Source: CAD feature listing. Evaluate the final solid. Frame: model axes, mm. Face numbers are marked on the shaded views. A direction names the side the tool comes from. Coordinates: 2 decimals unless noted, no trailing zeros. Loops run counter-clockwise (first coordinate to the right, second up) from the corner with the lowest first, then second, coordinate; pieces in that order, holes last. Notation, with made-up numbers: (-24.5, -35.75) - (14.5, -35.75) arc R19 ccw to (14.5, -23.75) - close; hole circle Ø1 at (-9.5, -7.5). An arc over 180 degrees is marked (long way). Use one line per item in the form item = value. Start each with the question number.
from build123d import *

# Parameters (mm, degrees)
BOSS_EXTRUDE1_DEPTH            = 3
BOSS_EXTRUDE1_DEPTH_BACK       = 12.8
SKETCH1_W                      = 6
SKETCH1_H                      = 6
SKETCH10_W                     = 6
SKETCH10_H                     = 3.25
BOSS_EXTRUDE2_DEPTH            = 0.75
CUT_EXTRUDE2_DEPTH             = 0.1
CUT_EXTRUDE2_DEPTH_BACK        = 1
CUT_EXTRUDE3_DEPTH             = 5.5
CUT_EXTRUDE3_DEPTH_BACK        = 6.5
SKETCH5_R                      = 4.45
CUT_EXTRUDE4_REACH             = 40.346
SKETCH7_R                      = 0.525
CUT_EXTRUDE4_DIRECTION_2_REACH = 40.346
SKETCH8_W                      = 3
SKETCH8_H                      = 6.75
CUT_EXTRUDE5_DEPTH             = 1
FILLET1_R                      = 3.5
FILLET1_R_2                    = 2.5
CUT_EXTRUDE7_DEPTH             = 39.676090947


with BuildPart() as part:
    # Sketch1 → Boss-Extrude1 (new, two sides: drawn at the far end of the back side and taken through both)
    with BuildSketch(Plane.XY.offset(-BOSS_EXTRUDE1_DEPTH_BACK)):
        with Locations((122, -33)):
            Rectangle(SKETCH1_W, SKETCH1_H)
    extrude(amount=BOSS_EXTRUDE1_DEPTH + BOSS_EXTRUDE1_DEPTH_BACK)

    # Sketch10 → Boss-Extrude2 (add)
    with BuildSketch(Plane(origin=(0, -30, 0), x_dir=(1, 0, 0), z_dir=(0, 1, 0))):
        with Locations((122, 11.175)):
            Rectangle(SKETCH10_W, SKETCH10_H)
    extrude(amount=BOSS_EXTRUDE2_DEPTH)

    # Sketch4 → Cut-Extrude2 (cut, two sides: drawn at the far end of the back side and taken through both)
    with BuildSketch(Plane.ZY.offset(-121.85).offset(-CUT_EXTRUDE2_DEPTH_BACK)):
        with BuildLine():
            Line((-11.776969868, -34.5), (-11.623346252, -34.5))
            ThreePointArc((-11.623346252, -34.5), (-10.835914556, -34.188123693), (-10.475580755, -33.421654477))
            Line((-10.475580755, -33.421654477), (-10.040343544, -26.45))
            Line((-10.040343544, -26.45), (-13.359649062, -26.45))
            Line((-13.359649062, -26.45), (-12.924738676, -33.421601422))
            ThreePointArc((-12.924738676, -33.421601422), (-12.564420934, -34.188105493), (-11.776969868, -34.5))
        make_face()
    extrude(amount=CUT_EXTRUDE2_DEPTH + CUT_EXTRUDE2_DEPTH_BACK, mode=Mode.SUBTRACT)

    # Sketch5 → Cut-Extrude3 (cut, two sides: drawn at the far end of the back side and taken through both)
    with BuildSketch(Plane(origin=(0, 0, -3.85), x_dir=(-1, 0, 0), z_dir=(0, 0, -1)).offset(-CUT_EXTRUDE3_DEPTH_BACK)):
        with Locations((-122.25, -26.35)):
            Circle(SKETCH5_R)
    extrude(amount=CUT_EXTRUDE3_DEPTH + CUT_EXTRUDE3_DEPTH_BACK, mode=Mode.SUBTRACT)

    # Cut-Extrude4: up to this face of the body (flat: up to its plane)
    cut_extrude4_end = Plane(part.part.faces().sort_by_distance((119, -32.915397223, -5.057298496))[0])
    # Sketch7 → Cut-Extrude4 (cut, up to the picked face)
    with BuildSketch(Plane(origin=(121.75, 0, 0), x_dir=(0, 0, -1), z_dir=(1, 0, 0)), mode=Mode.PRIVATE) as cut_extrude4_sk1:
        with Locations(Location((11.7, -33.35, 0), (0, 0, 90))):
            Circle(SKETCH7_R)
    cut_extrude4_tool1 = split(extrude(cut_extrude4_sk1.sketch, amount=-CUT_EXTRUDE4_REACH, mode=Mode.PRIVATE), bisect_by=cut_extrude4_end, keep=Keep.BOTH, mode=Mode.PRIVATE)
    # Sketch7 → Cut-Extrude4 (cut, up to the picked face)
    with BuildSketch(Plane(origin=(121.75, 0, 0), x_dir=(0, 0, -1), z_dir=(1, 0, 0)), mode=Mode.PRIVATE) as cut_extrude4_sk2:
        with Locations(Location((11.7, -30.35, 0), (0, 0, 90))):
            Circle(SKETCH7_R)
    cut_extrude4_tool2 = split(extrude(cut_extrude4_sk2.sketch, amount=-CUT_EXTRUDE4_REACH, mode=Mode.PRIVATE), bisect_by=cut_extrude4_end, keep=Keep.BOTH, mode=Mode.PRIVATE)
    add(cut_extrude4_tool1.solids().sort_by(Axis((121.75, -33.35, -11.7), (-1, 0, 0)))[0], mode=Mode.SUBTRACT)
    add(cut_extrude4_tool2.solids().sort_by(Axis((121.75, -30.35, -11.7), (-1, 0, 0)))[0], mode=Mode.SUBTRACT)

    # Cut-Extrude4 direction 2: up to this face of the body (flat: up to its plane)
    cut_extrude4_direction_2_end = Plane(part.part.faces().sort_by_distance((125, -32.915397223, -5.057298496))[0])
    # Sketch7 → Cut-Extrude4 direction 2 (cut, up to the picked face)
    with BuildSketch(Plane(origin=(121.75, 0, 0), x_dir=(0, 0, -1), z_dir=(1, 0, 0)), mode=Mode.PRIVATE) as cut_extrude4_direction_2_sk1:
        with Locations(Location((11.7, -33.35, 0), (0, 0, 90))):
            Circle(SKETCH7_R)
    cut_extrude4_direction_2_tool1 = split(extrude(cut_extrude4_direction_2_sk1.sketch, amount=CUT_EXTRUDE4_DIRECTION_2_REACH, mode=Mode.PRIVATE), bisect_by=cut_extrude4_direction_2_end, keep=Keep.BOTH, mode=Mode.PRIVATE)
    # Sketch7 → Cut-Extrude4 direction 2 (cut, up to the picked face)
    with BuildSketch(Plane(origin=(121.75, 0, 0), x_dir=(0, 0, -1), z_dir=(1, 0, 0)), mode=Mode.PRIVATE) as cut_extrude4_direction_2_sk2:
        with Locations(Location((11.7, -30.35, 0), (0, 0, 90))):
            Circle(SKETCH7_R)
    cut_extrude4_direction_2_tool2 = split(extrude(cut_extrude4_direction_2_sk2.sketch, amount=CUT_EXTRUDE4_DIRECTION_2_REACH, mode=Mode.PRIVATE), bisect_by=cut_extrude4_direction_2_end, keep=Keep.BOTH, mode=Mode.PRIVATE)
    add(cut_extrude4_direction_2_tool1.solids().sort_by(Axis((121.75, -33.35, -11.7), (1, 0, 0)))[0], mode=Mode.SUBTRACT)
    add(cut_extrude4_direction_2_tool2.solids().sort_by(Axis((121.75, -30.35, -11.7), (1, 0, 0)))[0], mode=Mode.SUBTRACT)

    # Sketch8 → Cut-Extrude5 (cut)
    with BuildSketch(Plane(origin=(125, 0, 0), x_dir=(0, 0, -1), z_dir=(1, 0, 0))):
        with Locations((11.3, -32.625)):
            Rectangle(SKETCH8_W, SKETCH8_H)
    extrude(amount=-CUT_EXTRUDE5_DEPTH, mode=Mode.SUBTRACT)

    # Fillet1
    # the kernel refuses this fillet: 3.5, 2.5 mm, written as the material it takes off along each edge
    with BuildSketch(Plane(origin=(132.75, -36, -12.8), x_dir=(0, 0, 1), z_dir=(-1, 0, 0))) as fillet1_piece_1:
        with BuildLine():
            CenterArc((FILLET1_R, FILLET1_R), FILLET1_R, 180, 90)
            Line((0, FILLET1_R), (0, 0))
            Line((0, 0), (FILLET1_R, 0))
        make_face()
    extrude(amount=22.5, mode=Mode.SUBTRACT)
    # the kernel refuses this fillet: 3.5, 2.5 mm, written as the material it takes off along each edge
    with BuildSketch(Plane(origin=(119, -23, -12.8), x_dir=(0, 0, 1), z_dir=(0, -1, 0))) as fillet1_2_piece_1:
        with BuildLine():
            CenterArc((FILLET1_R_2, -FILLET1_R_2), FILLET1_R_2, 90, 90)
            Line((0, -FILLET1_R_2), (0, 0))
            Line((0, 0), (FILLET1_R_2, 0))
        make_face()
    extrude(amount=15.75, mode=Mode.SUBTRACT)

    # Sketch12 → Cut-Extrude7 (cut, through all)
    with BuildSketch(Plane.ZY.offset(-119)):
        Polygon((-6.404787377, -36), (-12.404787377, -34.227808088), (-12.404787377, -36), align=None)
    extrude(amount=-CUT_EXTRUDE7_DEPTH, mode=Mode.SUBTRACT)


solid = part.part
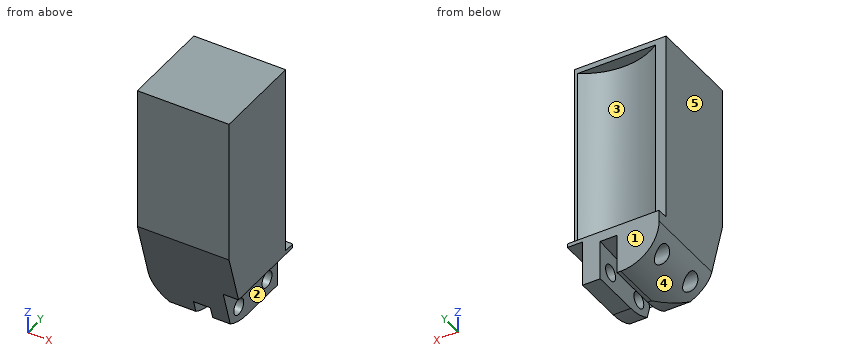
(1) Cut plane D-D, the plane z = -3.75. Output: boundary loops of the cut face in (x, y).
(2) Mould query, pull axis Z, two halves, no side actions, for the marked faces 3, 4 and 5. Classes: +Z half, -Z half, draft (parallel to the pull), parting line (faces both ways), or undercut.
(3) Access query for the marked faces 1 and 2. Directions: +Z, -Z, +X, -X, +Y, -Y. A direction counts if a zero-diameter tool reaches every point of the face in a straight line with its end or side. Return the directions, or none.
(4) Contact query for flat-ended pins moving along their axis: pin 1 (1.4 mm diameter, centred on y = -33.35, z = -11.7, fed in from +X); pin 2 (1.7 mm diameter, centred on y = -30.35, z = -11.7, fed in from -X); pin 3 (0.8 mm diameter, centred on y = -33.35, z = -11.7, fed in from +X); pin 4 (1 mm diameter, centred on x = 123.5, z = -8, fed in from +Y). Output: stop coordinate, or through.
(5) Cut plane B-B, the plane x = 120.25. Output: boundary loops of the cut face in (y, z) (3 decimals), plus the area to 3 significant figures.
(6) Material intervals for line 1 (Z direction, x = 123.6, y = -30.35) (3 decimals); line 2 (Y direction, x = 123.35, z = -11.7) (3 decimals); line 3 (Z direction, x = 120.65, y = -30.35) (3 decimals), sorted ascending.
(7) Cut plane A-A, the plane y = -33. Output: boundary loops of the cut face in (x, z), plus the area to 3 significant figures.
(8) Cut plane C-C, the plane y = -30.35. Output: boundary loops of the cut face in (x, z) (3 decimals).
Recorded:
q1.outline = (119, -36) - (125, -36) - (125, -30) - (124.8, -30) arc R4.45 cw to (119.7, -30) - (119, -30) - close
q2.face_3 = undercut
q2.face_4 = -Z half
q2.face_5 = draft
q3.face_1 = +Z, -Z, +X, -X, +Y
q3.face_2 = -Z, +X, +Y, -Y
q4.pin_1 = 124
q4.pin_2 = 119.06
q4.pin_3 = through
q4.pin_4 = -30.44
q5.outline = (-36, -6.405) - (-34.249, -12.331) arc R3.5 ccw to (-33.994, -12.465) - (-29.25, -12.465) - (-29.25, -9.55) - (-30, -9.55) - (-30, -9.35) - (-30.325, -9.35) - (-30.325, 2.65) - (-30, 2.65) - (-30, 3) - (-36, 3) - close; hole circle Ø1.05 at (-33.35, -11.7); hole circle Ø1.05 at (-30.35, -11.7)
q5.area = 83.9 mm²
q6.line_1 = -12.8 to -12.225, -11.175 to -9.35, 2.65 to 3
q6.line_2 = -34.436 to -33.875, -32.825 to -30.875, -29.825 to -29.25
q6.line_3 = -12.651 to -12.225, -11.175 to -9.35, 2.65 to 3
q7.outline = (119, -10.3) arc R2.5 ccw to (119.21, -11.31) - (121.75, -11.31) - (121.75, -10.45) - (122.85, -10.45) - (122.85, -11.31) - (124, -11.31) - (124, -9.8) - (125, -9.8) - (125, 3) - (119, 3) - close; (119.76, -12.09) arc R2.5 ccw to (121.08, -12.76) - (121.75, -12.76) - (121.75, -12.09) - close; (122.85, -12.76) - (124, -12.76) - (124, -12.09) - (122.85, -12.09) - close
q7.area = 85.1 mm²
q8.outline = (119, -10.3) arc R2.5 ccw to (119.158, -11.175) - (121.75, -11.175) - (121.75, -10.284) - (122.85, -10.284) - (122.85, -11.175) - (124, -11.175) - (124, -9.8) - (125, -9.8) - (125, 3) - (119, 3) - close; (119.905, -12.225) arc R2.5 ccw to (121.5, -12.8) - (121.75, -12.8) - (121.75, -12.225) - close; (122.85, -12.8) - (124, -12.8) - (124, -12.225) - (122.85, -12.225) - close; hole (120.3, -9.35) - (124.2, -9.35) - (124.2, 2.65) - (120.3, 2.65) - close
